Source: CAD feature listing. Evaluate the final solid. Frame: model axes, mm. Face numbers are marked on the shaded views. A direction names the side the tool comes from. Give positions to 0.01 mm unless a question says otherwise; leave off trailing zeros. Write each loop counter-clockwise with the first axis right and the second up, starting at its lowest first coordinate (ties: lowest second). Pieces come first, ordered by that corner, then holes. Notation, with made-up numbers: (-11, 18) - (28, 18) arc R18 ccw to (28, 36) - close; hole circle Ø6 at (34, 1.25). An arc over 180 degrees is marked (long way). One line per question, with ' | ' between items. Start each with the question number.
(1) Section A-A, the plane y = 12.7. Return loops of the section in (x, z), plus the area to 3 significant figures.
(2) Ray query, line 1 (Z direction, x = -12.7, y = 3.35); line 2 (Y direction, x = -3.1, z = 0); line 3 (Y direction, x = -9.75, z = 4.5). Return the intervals inside material, ascending. Write a range as [from, to].
(3) Section D-D, the plane z = 8.5. Return loops of the section in (x, y).
(4) Pin query (flat end, axial travel): pin 1 (6 mm diameter, centred on y = 18, z = 0.5, fed in from +X); pin 2 (6 mm diameter, centred on x = -14.5, z = -7, fed in from +Y); pin 3 (6 mm diameter, centred on y = 17, z = 3, fed in from -X); pin 4 (1 mm diameter, centred on x = -20.5, y = 5.5, fed in from -Z). Return the tip coordinate at first contact, or that it passes through.
(5) Access query for the marked faces 1 and 2. Directions: +Z, -Z, +X, -X, +Y, -Y. A direction counts if a zero-diameter tool reaches every point of the face in a straight line with its end or side. Return the directions, or none.
(6) Section B-B, the plane x = -12.7. Return loops of the section in (y, z).
(7) Section C-C, the plane z = 0. Return loops of the section in (x, y).
(8) Draft query along Z for the marked faces 3, 4, 5 and 6. Return one class per face: +Z half, -Z half, draft (parallel to the pull), parting line (faces both ways), or undercut.
```python
from build123d import *

# Parameters (mm, degrees)
EXTRUDE1_DEPTH     = 11.1125
SKETCH2_R          = 3.5687
CUT_EXTRUDE1_DEPTH = 5.7752
SKETCH3_R          = 3.5687
CUT_EXTRUDE2_DEPTH = 5.7752


with BuildPart() as part:
    # Sketch1 → Extrude1 (new body, symmetric)
    with BuildSketch(Plane.XY):
        with BuildLine():
            Line((0, 0), (0, 25.4))
            ThreePointArc((0, 25.4), (-3.376576302, 24.001376302), (-4.7752, 20.6248))
            Line((-4.7752, 20.6248), (-4.7752, 8.3566))
            ThreePointArc((-4.7752, 8.3566), (-5.824167774, 5.824167774), (-8.3566, 4.7752))
            Line((-8.3566, 4.7752), (-20.6248, 4.7752))
            ThreePointArc((-20.6248, 4.7752), (-24.001376302, 3.376576302), (-25.4, 0))
            Line((-25.4, 0), (0, 0))
        make_face()
    extrude(amount=EXTRUDE1_DEPTH, both=True)

    # Sketch2 → Cut-Extrude1 (cut, through all)
    with BuildSketch(Plane(origin=(0, 4.7752, 0), x_dir=(1, 0, 0), z_dir=(0, 1, 0))):
        with Locations((-12.7, 0)):
            Circle(SKETCH2_R)
    extrude(amount=-CUT_EXTRUDE1_DEPTH, mode=Mode.SUBTRACT)

    # Sketch3 → Cut-Extrude2 (cut, through all)
    with BuildSketch(Plane.ZY.offset(4.7752)):
        with Locations((0, 12.7)):
            Circle(SKETCH3_R)
    extrude(amount=-CUT_EXTRUDE2_DEPTH, mode=Mode.SUBTRACT)


solid = part.part
```
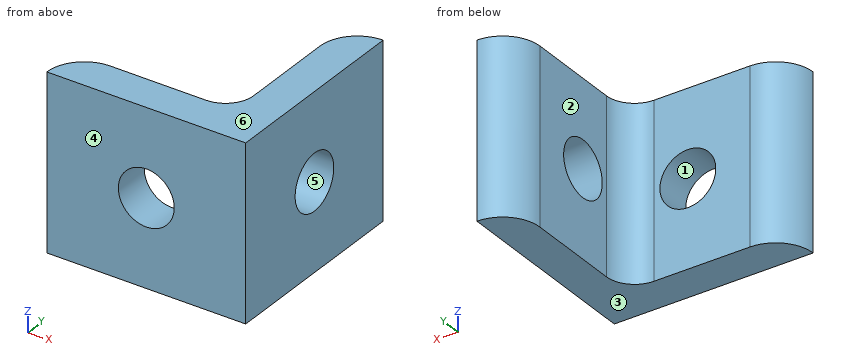
Check sheet entries:
1) outline: (-4.78, -11.11) - (0, -11.11) - (0, -3.57) - (-4.78, -3.57) - close; (-4.78, 3.57) - (0, 3.57) - (0, 11.11) - (-4.78, 11.11) - close | area: 72.0 mm²
2) line 1: [-11.11, -3.57], [3.57, 11.11] | line 2: [0, 9.13], [16.27, 24.26] | line 3: [0, 4.78]
3) outline: (-25.4, 0) - (0, 0) - (0, 25.4) arc R4.78 ccw to (-4.78, 20.62) - (-4.78, 8.36) arc R3.58 cw to (-8.36, 4.78) - (-20.62, 4.78) arc R4.78 ccw to start
4) pin 1: x = 0 | pin 2: y = 4.78 | pin 3: x = -4.78 | pin 4: through
5) face 1: +Y, -Y | face 2: +Z, -Z, -X, +Y
6) outline: (0, -11.11) - (4.78, -11.11) - (4.78, -3.57) - (0, -3.57) - close; (0, 3.57) - (4.78, 3.57) - (4.78, 11.11) - (0, 11.11) - close
7) outline: (-25.4, 0) - (-16.27, 0) - (-16.27, 4.78) - (-20.62, 4.78) arc R4.78 ccw to start; (-9.13, 0) - (0, 0) - (0, 9.13) - (-4.78, 9.13) - (-4.78, 8.36) arc R3.58 cw to (-8.36, 4.78) - (-9.13, 4.78) - close; (-4.78, 16.27) - (0, 16.27) - (0, 25.4) arc R4.78 ccw to (-4.78, 20.62) - close
8) face 3: -Z half | face 4: draft | face 5: undercut | face 6: +Z half
